Source: CAD feature listing. Evaluate the final solid. Frame: model axes, mm. A direction names the side the tool comes from. Give positions to 0.01 mm unless a question says otherwise; leave off trailing zeros. Order: outer loops, then holes, each group sorted by start corner. A loop starts at its lowest first (then second) coordinate and runs counter-clockwise, first axis right, second up. Notation, with made-up numbers: (-4.75, 56.5) - (17.25, 56.5) arc R26 cw to (17.25, 75.5) - close; hole circle Ø2 at (-8, 82.25). An arc over 180 degrees is marked (long way). Use CSV: the item, a comma, the result in double quotes.
```python
from build123d import *

# Parameters (mm, degrees)
SKETCH1_W          = 203.2
SKETCH1_H          = 3.175
REVOLVE1_ANGLE     = 90
SKETCH2_W          = 203.2
SKETCH2_H          = 3.175
CUT_EXTRUDE1_DEPTH = 313.926814527
SKETCH3_W          = 165.1
SKETCH3_H          = 101.6
CUT_EXTRUDE2_DEPTH = 312.230984359


# Read off the part's stored shape, not the designer's step: #10 Clearance Hole1
with BuildPart() as part:
    # Sketch1 → Revolve1 (revolve)
    with BuildSketch(Plane.XY):
        with Locations((-101.6, 19.434848485)):
            Rectangle(SKETCH1_W, SKETCH1_H)
    revolve(axis=Axis((-168.467424242, -147.252651515, 0), (-1, 0, 0)), revolution_arc=REVOLVE1_ANGLE)

    # Sketch2 → Cut-Extrude1 (cut, through all)
    with BuildSketch(Plane(origin=(0, -147.252651515, 0), x_dir=(-1, 0, 0), z_dir=(0, -1, 0))):
        with Locations((101.6, 166.6875)):
            Rectangle(SKETCH2_W, SKETCH2_H)
    extrude(amount=-CUT_EXTRUDE1_DEPTH, mode=Mode.SUBTRACT)

    # Sketch3 → Cut-Extrude2 (cut, through all)
    with BuildSketch(Plane.XZ.offset(147.252651515)):
        with Locations((-101.6, -114.3)):
            Rectangle(SKETCH3_W, SKETCH3_H)
    extrude(amount=-CUT_EXTRUDE2_DEPTH, mode=Mode.SUBTRACT)

    # #10 Clearance Hole1 outline → #10 Clearance Hole1 (revolve, cut)
    with BuildSketch(Plane(origin=(-63.5, -15.166166065, -37.2189581), x_dir=(1, 0, 0), z_dir=(0, 0.3773584905660381, 0.9260672597590962))):
        Polygon((2.5527, 30.49567621), (0, 30.49567621), (0, 27.797130409), (2.187572038, 27.797130409), (2.5527, 28.016521422), align=None)
    revolve(axis=Axis((-63.5, -15.166166065, -37.2189581), (0, 0.9260672597590962, -0.3773584905660381)), mode=Mode.SUBTRACT)

    # 10 Clearance Hole1 2 outline → 10 Clearance Hole1 2 (revolve, cut)
    with BuildSketch(Plane(origin=(-114.3, -15.166166065, -37.2189581), x_dir=(1, 0, 0), z_dir=(0, 0.3773584905660381, 0.9260672597590962))):
        Polygon((0, 30.49567621), (0, 27.797130409), (2.187572038, 27.797130409), (2.5527, 28.016521422), (2.5527, 30.49567621), align=None)
    revolve(axis=Axis((-114.3, -15.166166065, -37.2189581), (0, 0.9260672597590962, -0.3773584905660381)), mode=Mode.SUBTRACT)


solid = part.part
```
Item 1: Set-up query: faces 4 (the flat face through (-114.34, 13.06, -48.76)), 5 (the flat face through (-203.2, -19, -107)). Return all of +Z, -Z, +X, -X, +Y, -Y with unobstructed straight access to the full face (end or side cutting, diameter ignored); none if empty.
Filled in:
face 4,"none"
face 5,"+Z, -Z, -X, +Y, -Y"
Item 2: Section A-A on z = -104.5. Return the cut outline in (x, y), then the cut area to 3 significant figures.
Filled in:
outline,"(-203.2, -19.43) - (-184.15, -19.43) - (-184.15, -15.36) - (-203.2, -15.36) - close; (-19.05, -19.43) - (0, -19.43) - (0, -15.36) - (-19.05, -15.36) - close"
area,"155 mm2"
Item 3: First-contact query: pin 1 (4 mm diameter, centred on x = -93, y = 6, fed in from -Z); pin 2 (2 mm diameter, centred on x = -166.5, z = -62, fed in from +Y); pin 3 (3 mm diameter, centred on x = -49.5, z = -40, fed in from -Y). Flat tips, straight axial feed; report the tip coordinate or a pass-through.
Filled in:
pin 1,"stops at z = -63.5"
pin 2,"stops at y = 9.58"
pin 3,"stops at y = 12.55"
Item 4: Section C-C on x = -137.5. Return the cut outline in (y, z) (3 decimals).
Filled in:
outline,"(5.147, -63.5) - (8.581, -63.5) arc R168.275 ccw to (21.022, 0) - (17.847, 0) arc R165.1 cw to start"
Item 5: Section D-D on z = -28. Return the cut outline in (x, y).
Filled in:
outline,"(-203.2, 15.46) - (0, 15.46) - (0, 18.68) - (-203.2, 18.68) - close"
Item 6: Section B-B on y = -88.5. Return the cut outline in (x, z), then the cut area to 3 significant figures.
Filled in:
outline,"(-203.2, -157.69) - (-184.15, -157.69) - (-184.15, -154.29) - (-203.2, -154.29) - close; (-19.05, -157.69) - (0, -157.69) - (0, -154.29) - (-19.05, -154.29) - close"
area,"129 mm2"
Item 7: Material intervals for line 1 (Y direction, x = -82, z = -54.5); line 2 (Z direction, x = -17.5, y = -52.5); line 3 (Z direction, x = -192, y = -103), sorted ascending. Write a range as from..to.
Filled in:
line 1,"y = 8.59..11.95"
line 2,"z = -139.06..-135.2"
line 3,"z = -162.35..-159.06"
Item 8: Mould query, pull axis Z, two halves, no side actions, for faces 1 (the flat face through (-194, -131, -165.1)), 2 (the flat face through (-19.05, -47, -133)), 3 (the flat face through (-63.54, 13.06, -48.76)). Classes: released by +Z, released by -Z, zero draft, split by the parting line, or undercut.
Filled in:
face 1,"released by -Z"
face 2,"zero draft"
face 3,"undercut"
